```python
from build123d import *

# Parameters (mm, degrees)
SKETCH1_W           = 31.75
SKETCH1_H           = 101.6
BOSS_EXTRUDE1_DEPTH = 31.75
SKETCH2_R           = 4.9609375
CUT_EXTRUDE1_DEPTH  = 112.079633597
SKETCH3_R           = 6.35
CUT_EXTRUDE2_DEPTH  = 112.079633597


with BuildPart() as part:
    # Sketch1 → Boss-Extrude1 (new body)
    with BuildSketch(Plane.XY):
        with Locations((15.875, 50.8)):
            Rectangle(SKETCH1_W, SKETCH1_H)
    extrude(amount=BOSS_EXTRUDE1_DEPTH)

    # Sketch2 → Cut-Extrude1 (cut, through all)
    with BuildSketch(Plane.XY.offset(31.75)):
        with Locations((15.875, 88.9)):
            Circle(SKETCH2_R)
        with Locations((15.875, 63.5)):
            Circle(SKETCH2_R)
    extrude(amount=-CUT_EXTRUDE1_DEPTH, mode=Mode.SUBTRACT)

    # Sketch3 → Cut-Extrude2 (cut, through all)
    with BuildSketch(Plane.ZY):
        with Locations((15.875, 15.875)):
            Circle(SKETCH3_R)
    extrude(amount=-CUT_EXTRUDE2_DEPTH, mode=Mode.SUBTRACT)


solid = part.part
```
The listing builds one solid part. Answer for the finished solid, in the listing's coordinates (mm). Coordinates: 2 decimals unless noted, no trailing zeros. Loops run counter-clockwise (first coordinate to the right, second up) from the corner with the lowest first, then second, coordinate; pieces in that order, holes last. Notation, with made-up numbers: M 28.25,-18.5 L 81.25,-18.5 A20 cw 81.25,5.5 Z; hole C 79.25,68.25 d3. An arc over 180 degrees is marked long. Answer as CSV lines item,"result". Start each with the question number.
(1) Given pin 1 (6 mm diameter, centred on y = 86.5, z = 19, fed in from -X); pin 2 (6 mm diameter, centred on x = 15.875, y = 88.9, fed in from -Z), each flat-ended and moving along its own axis, determine where each tip first touches the part or whether it passes through.
(2) The part is cut by section A-A (y = 88.9). Give the vertices of the cut face in (x, z), and give its area (3 significant figures).
(3) The mould has two halves that part along Y. Classify faces 1 (the flat face through (16, 0, 16)), 2 (the flat face through (16, 101.6, 16)), 3 (the cylindrical face through (15.653, 10.241, 18.805)): pulls with the +Y half, pulls with the -Y half, needs draft (parallel to the pull), parting line crosses it, or undercut.
(4) The part is cut by section C-C (x = 15.5). Give the vertices of the cut face in (y, z) (3 decimals), and give its area (3 significant figures).
(5) The part is cut by section D-D (z = 3.5). Give the vertices of the cut face in (x, y) (3 decimals).
(6) The part is cut by section B-B (z = 12). Give the vertices of the cut face in (x, y) (3 decimals), and give its area (3 significant figures).
(7) Find the intervals of material crossed by L1, parallel to Z at x = 13.5, y = 15.5; L2, parallel to Y at x = 17.5, z = 21.5; L3, parallel to Z at x = 5, y = 13, in increasing order. Write a range as [from, to].
Determined:
1,pin 1,"x = 0"
1,pin 2,"through"
2,outline,"M 0,0 L 10.91,0 L 10.91,31.75 L 0,31.75 Z; M 20.84,0 L 31.75,0 L 31.75,31.75 L 20.84,31.75 Z"
2,area,"693 mm2"
3,face 1,"pulls with the -Y half"
3,face 2,"pulls with the +Y half"
3,face 3,"undercut"
4,outline,"M 0,0 L 58.553,0 L 58.553,31.75 L 0,31.75 Z; M 68.447,0 L 83.953,0 L 83.953,31.75 L 68.447,31.75 Z; M 93.847,0 L 101.6,0 L 101.6,31.75 L 93.847,31.75 Z; hole C 15.875,15.875 d12.7"
4,area,"2,470 mm2"
5,outline,"M 0,0 L 31.75,0 L 31.75,101.6 L 0,101.6 Z; hole C 15.875,63.5 d9.922; hole C 15.875,88.9 d9.922"
6,outline,"M 0,0 L 31.75,0 L 31.75,10.844 L 0,10.844 Z; M 0,20.906 L 31.75,20.906 L 31.75,101.6 L 0,101.6 Z; hole C 15.875,63.5 d9.922; hole C 15.875,88.9 d9.922"
6,area,"2,750 mm2"
7,L1,"[0, 9.54], [22.21, 31.75]"
7,L2,"[0, 12.93], [18.82, 58.81], [68.19, 84.21], [93.59, 101.6]"
7,L3,"[0, 10.21], [21.54, 31.75]"
